```python
from build123d import *

# Parameters (mm, degrees)
ESQUISSE1_W             = 247
ESQUISSE1_H             = 267
BOSS_EXTRU_1_DEPTH      = 3
ESQUISSE3_R             = 6.5
ESQUISSE3_R_2           = 12.5
ENL_V_MAT_EXTRU_2_DEPTH = 3
ESQUISSE4_W             = 120
ESQUISSE4_H             = 25
ENL_V_MAT_EXTRU_3_DEPTH = 10
CONG_1_R                = 30
CONG_2_R                = 5


with BuildPart() as part:
    # Esquisse1 → Boss.-Extru.1 (new body)
    with BuildSketch(Plane.XY):
        Rectangle(ESQUISSE1_W, ESQUISSE1_H)
    extrude(amount=BOSS_EXTRU_1_DEPTH)

    # Esquisse3 → Enlèv. mat.-Extru.2 (cut)
    with BuildSketch(Plane(origin=(0, 0, 0), x_dir=(-1, 0, 0), z_dir=(0, 0, -1))):
        with Locations((-59.966662183, -113.5)):
            Circle(ESQUISSE3_R)
        with Locations((-16.5, -101.85314297)):
            Circle(ESQUISSE3_R_2)
        with Locations((26.966662183, -90.206285941)):
            Circle(ESQUISSE3_R)
    extrude(amount=-ENL_V_MAT_EXTRU_2_DEPTH, mode=Mode.SUBTRACT)

    # Esquisse4 → Enlèv. mat.-Extru.3 (cut)
    with BuildSketch(Plane(origin=(0, 0, 0), x_dir=(-1, 0, 0), z_dir=(0, 0, -1))):
        with Locations((66.5, -19)):
            Rectangle(ESQUISSE4_W, ESQUISSE4_H)
    extrude(amount=-ENL_V_MAT_EXTRU_3_DEPTH, mode=Mode.SUBTRACT)

    # Congé1
    cong_1_edges = [part.edges().sort_by_distance(p)[0] for p in [
        (123.5, -133.5, 1.5),
        (-123.5, -133.5, 1.5),
    ]]
    fillet(cong_1_edges, radius=CONG_1_R)

    # Congé2
    cong_2_edges = [part.edges().sort_by_distance(p)[0] for p in [
        (-6.5, -31.5, 1.5),
        (-6.5, -6.5, 1.5),
    ]]
    fillet(cong_2_edges, radius=CONG_2_R)


solid = part.part
```
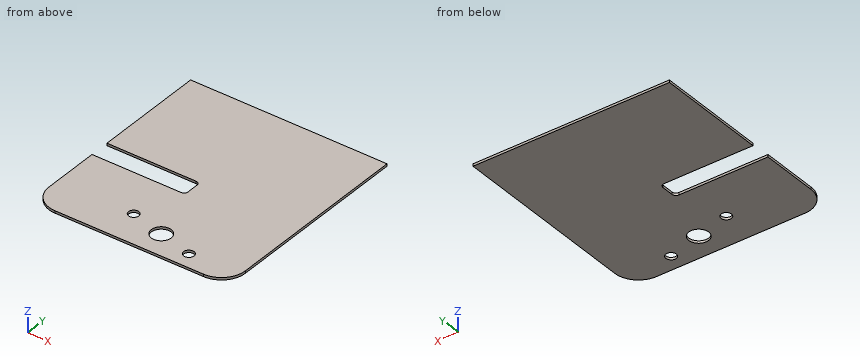
For this review, take the finished solid that the model builds, in its own axes (mm). Round coordinates to 2 decimals unless told otherwise and drop trailing zeros. Loops run counter-clockwise (first coordinate to the right, second up) from the corner with the lowest first, then second, coordinate; pieces in that order, holes last.
(1) We need section A-A (x = 16.5). Give the boundary of the cut face in (y, z).
Returned:
outline: (-133.5, 0) - (-114.35, 0) - (-114.35, 3) - (-133.5, 3) - close; (-89.35, 0) - (133.5, 0) - (133.5, 3) - (-89.35, 3) - close
(2) We need section B-B (z = 1.8). Give the boundary of the cut face in (x, y), plus the area to 3 significant figures.
Returned:
outline: (-123.5, -103.5) arc R30 ccw to (-93.5, -133.5) - (93.5, -133.5) arc R30 ccw to (123.5, -103.5) - (123.5, 133.5) - (-123.5, 133.5) - (-123.5, -6.5) - (-11.5, -6.5) arc R5 cw to (-6.5, -11.5) - (-6.5, -26.5) arc R5 cw to (-11.5, -31.5) - (-123.5, -31.5) - close; hole circle Ø13 at (-26.97, -90.21); hole circle Ø25 at (16.5, -101.85); hole circle Ø13 at (59.97, -113.5)
area: 61,900 mm2
(3) We need section C-C (x = -104). Give the boundary of the cut face in (y, z), plus the area to 3 significant figures.
Returned:
outline: (-131.6, 0) - (-31.5, 0) - (-31.5, 3) - (-131.6, 3) - close; (-6.5, 0) - (133.5, 0) - (133.5, 3) - (-6.5, 3) - close
area: 720 mm2
(4) Wall thickness on line 1 along Y through (x, z) = (16.5, 0.8); line 2 along Y through (x, z) = (-19.5, 0.65); line 3 along Y through (x, z) = (-28, 1.3): over which ranges is each line inside the solid? List them lowest first.
Returned:
line 1: y = -133.5 to -114.35, -89.35 to 133.5
line 2: y = -133.5 to -31.5, -6.5 to 133.5
line 3: y = -133.5 to -96.62, -83.79 to -31.5, -6.5 to 133.5
